Work out the finished part from the listing and answer in its coordinate system (mm). Face numbers are marked on the shaded views. A direction names the side the tool comes from. Coordinates: 2 decimals unless noted, no trailing zeros. Write each loop counter-clockwise with the first axis right and the second up, starting at its lowest first coordinate (ties: lowest second). Pieces come first, ordered by that corner, then holes. Notation, with made-up numbers: (4.25, 8) - (37.25, 8) arc R23 ccw to (37.25, 21) - close; hole circle Ø8 at (33.25, 62.25). An arc over 180 degrees is marked (long way). Use a Markdown table: item, result. Add a question column.
(1) Find the intervals of material crossed by line 1 (Y direction, x = 39.5, z = 17.5); line 2 (X direction, y = 50, z = 0.5) (3 decimals); line 3 (Z direction, x = 99, y = -22) (3 decimals), in increasing order. Write a range as from..to.
(2) The part is cut by section B-B, the plane y = -30. Give the vertices of the cut face in (x, z) (3 decimals), then the cut area to 3 significant figures.
(3) For a pull along X with two mould halves and no side action, classify the marked faces 1, 2 and 3 as released by +X, released by -X, zero draft, split by the parting line, or undercut.
(4) A tool of negligible diameter and unlimited length cuts with its end or side. For the marked faces 4, 5, 6 and 7, from which of +Z, -Z, +X, -X, +Y, -Y can it reach the whole face along a straight path? Write none if from no direction.
(5) The part is cut by section A-A, the plane x = 73. Give the vertices of the cut face in (y, z) (3 decimals), then the cut area to 3 significant figures.
(6) Given pin 1 Ø4 at (y, z) = (-17, 35.5) entering from -X; pin 2 Ø17 at (x, z) = (39.5, 36.5) entering from -Y; pin 3 Ø18 at (x, y) = (90.5, -11) entering from -Z, each flat-ended and moving along its own axis, determine where each tip first touches the part or whether it passes through.
from build123d import *

# Parameters (mm, degrees)
F1_DEPTH = 63.5
F0_W     = 25.4
F0_H     = 4.7752
F0_H_2   = 19.05
F0_H_3   = 4.7498
F2_DEPTH = 22.606


with BuildPart() as f1:
    # F0 (on Front) → F1 (new body, symmetric)
    with BuildSketch(Plane.XZ):
        Polygon((-41.275, -9.525), (41.275, -9.525), (41.275, 9.525), (22.225, 9.525), (-41.275, 9.525), align=None)
    extrude(amount=F1_DEPTH, both=True)

    # F0 (on Front) → F2 (join)
    with BuildSketch(Plane.XZ):
        Polygon((-41.275, -9.525), (41.275, -9.525), (41.275, 9.525), (22.225, 9.525), (-41.275, 9.525), align=None)
        with BuildLine():
            Line((22.225, 9.525), (41.275, 9.525))
            Line((41.275, 9.525), (41.275, 27.0002))
            ThreePointArc((41.275, 27.0002), (45.9246798487, 38.2255201513), (57.15, 42.8752))
            Line((57.15, 42.8752), (60.325, 42.8752))
            Line((60.325, 42.8752), (60.325, 61.9252))
            Line((60.325, 61.9252), (57.15, 61.9252))
            add(Edge.make_bspline(
                [(56.6150518391, 61.9211028444), (56.7937815954, 61.9227744977), (56.9721001461, 61.924139948), (57.15, 61.9252)],
                knots=[110.9922728255, 110.9922728255, 110.9922728255, 110.9922728255, 111.5045361635, 111.5045361635, 111.5045361635, 111.5045361635], degree=3))
            ThreePointArc((56.6150518391, 61.9211028444), (32.2658816761, 51.5060417574), (22.225, 27.0002))
            Line((22.225, 27.0002), (22.225, 9.525))
        make_face()
        with BuildLine():
            add(Edge.make_bspline(
                [(-41.275, 9.525), (-40.1402965099, 46.8216899359), (17.8896143528, 61.5589051427), (56.6150518391, 61.9211028444)],
                knots=[0, 0, 0, 0, 110.9922728255, 110.9922728255, 110.9922728255, 110.9922728255], degree=3))
            Line((-41.275, 9.525), (22.225, 9.525))
            Line((22.225, 9.525), (22.225, 27.0002))
            ThreePointArc((22.225, 27.0002), (32.2658816761, 51.5060417574), (56.6150518391, 61.9211028444))
        make_face()
        with BuildLine():
            ThreePointArc((57.15, 61.9252), (56.8825180747, 61.9241756961), (56.6150518391, 61.9211028444))
            add(Edge.make_bspline(
                [(56.6150518391, 61.9211028444), (56.7937815954, 61.9227744977), (56.9721001461, 61.924139948), (57.15, 61.9252)],
                knots=[110.9922728255, 110.9922728255, 110.9922728255, 110.9922728255, 111.5045361635, 111.5045361635, 111.5045361635, 111.5045361635], degree=3))
        make_face()
        with Locations((73.025, 40.4876)):
            Rectangle(F0_W, F0_H)
        with Locations((73.025, 52.4002)):
            Rectangle(F0_W, F0_H_2)
        with Locations((73.025, 64.3001)):
            Rectangle(F0_W, F0_H_3)
        Polygon((85.725, 61.9252), (85.725, 42.8752), (85.725, 38.1), (111.125, 38.1), (111.125, 66.675), (85.725, 66.675), align=None)
    extrude(amount=F2_DEPTH)


solid = f1.part
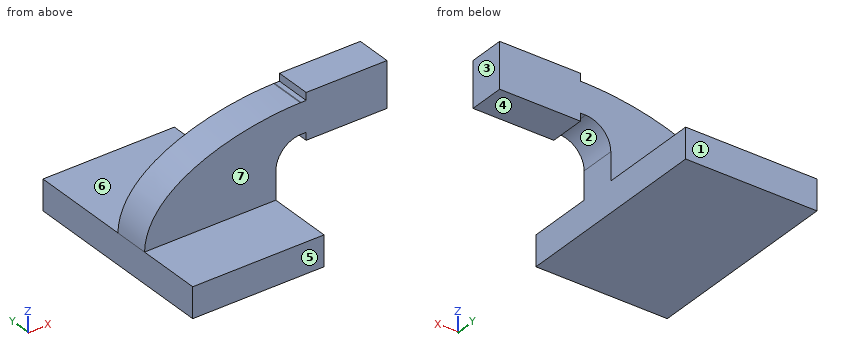
Model answer:
| question | item | result |
|---|---|---|
| 1 | line 1 | -22.61..0 |
| 1 | line 2 | -41.275..41.275 |
| 1 | line 3 | 38.1..66.675 |
| 2 | outline | (-41.275, -9.525) - (41.275, -9.525) - (41.275, 9.525) - (-41.275, 9.525) - close |
| 2 | area | 1,570 mm^2 |
| 3 | face 1 | zero draft |
| 3 | face 2 | undercut |
| 3 | face 3 | released by +X |
| 4 | face 4 | -Z, +X, +Y, -Y |
| 4 | face 5 | +Z, -Z, +X, -X, -Y |
| 4 | face 6 | +Z, +X, -X, +Y |
| 4 | face 7 | +Z, +X, -X, -Y |
| 5 | outline | (-22.606, 38.1) - (0, 38.1) - (0, 66.675) - (-22.606, 66.675) - close |
| 5 | area | 646 mm^2 |
| 6 | pin 1 | x = -30.85 |
| 6 | pin 2 | y = -22.61 |
| 6 | pin 3 | z = 38.1 |
